For this review, take the finished solid that the model builds, in its own axes (mm). Give positions to 0.01 mm unless a question says otherwise; leave off trailing zeros. Write each loop counter-clockwise with the first axis right and the second up, starting at its lowest first coordinate (ties: lowest second). Pieces come first, ordered by that corner, then holes. Notation, with made-up numbers: (19.25, -3.5) -> (57.25, -3.5) arc R20 ccw to (57.25, 19.5) -> close; hole circle Ø3 at (57.5, 17). An arc over 180 degrees is marked (long way). Write item = value, one per line.
```python
from build123d import *

# Parameters (mm, degrees)
FASE1_SIZE = 0.1


with BuildPart() as part:
    # Skizze2 → Rotation1 (revolve)
    with BuildSketch(Plane(origin=(0, 0, 0), x_dir=(0, 0, -1), z_dir=(1, 0, 0)), mode=Mode.PRIVATE) as rotation1_sk:
        Polygon((-1, 2), (1, 2), (1, 2.5), (0.75, 2.5), (0.75, 3.4), (1, 3.4), (1, 4), (-1, 4), (-1, 3.4), (-0.75, 3.4), (-0.75, 2.5), (-1, 2.5), align=None)
    revolve(rotation1_sk.sketch.rotate(Axis((0, 0, 11.845846522), (0, 0, -1)), 90), axis=Axis((0, 0, 11.845846522), (0, 0, -1)))

    # Fase1
    fase1_edges = [part.edges().sort_by_distance(p)[0] for p in [
        (-4, 0, 1),
        (-4, 0, -1),
        (-2, 0, -1),
        (-2, 0, 1),
    ]]
    chamfer(fase1_edges, length=FASE1_SIZE)


solid = part.part
```
(1) Take a section at C-C (z = -0.4). Write out the cut boundary in (x, y).
Answers below:
outline = circle Ø8 at (0, 0); hole circle Ø4 at (0, 0)
(2) The part is to be moulded in two halves that separate along X. For faces 1 (the face through (-2, -2, 0.75)), 2 (the face through (2, -2, -0.75)), 3 (the face through (-0.867, 3.905, 0.013)), 4 (the face through (2, -3, 1)), say which applies: released by +X, released by -X, zero draft, split by the parting line, or undercut.
Answers below:
face_1 = undercut
face_2 = undercut
face_3 = split by the parting line
face_4 = zero draft
(3) To check wall thickness, follow probe 1 along Y at (x, z) = (0, -0.85); probe 2 along Y at (x, z) = (0, 0.45); probe 3 along Z at (x, y) = (-0.75, -3.25). State the ranges of each line that lie inside material, in increasing order.
Answers below:
probe_1 = -4 to -3.4, -2.5 to -2, 2 to 2.5, 3.4 to 4
probe_2 = -4 to -2, 2 to 4
probe_3 = -0.75 to 0.75
